Build history of the part. All positions in model axes, mm. Face numbers are marked on the shaded views. A direction names the side the tool comes from. Give positions to 0.01 mm unless a question says otherwise; leave off trailing zeros. Loops run counter-clockwise (first coordinate to the right, second up) from the corner with the lowest first, then second, coordinate; pieces in that order, holes last. Notation, with made-up numbers: (25.25, 39) - (29.25, 39) arc R20 cw to (29.25, 64) - close; hole circle Ø9 at (64.25, 30). An arc over 180 degrees is marked (long way). Return JSON: item names as keys, results as strings. Group by question number.
1) Slice it at A-A (z = 13.75). List the corners of the cut face in (x, y).
2) Slice it at D-D (y = 14). List the corners of the cut face in (x, z), and give its area (3 significant figures).
3) Slice it at C-C (y = -11). List the corners of the cut face in (x, z), and give its area (3 significant figures).
4) Drop flat-ended pins along their axis: pin 1 (6 mm diameter, centred on x = 0, z = 11, fed in from +Y); pin 2 (4 mm diameter, centred on x = 34.5, z = 5, fed in from -Y); pin 3 (7 mm diameter, centred on x = 28.5, z = 5.5, fed in from +Y). Give the stop position or say it passes through.
5) Drill centre lines: probe 1 along Y at (x, z) = (34.5, 2.5); probe 2 along X at (y, z) = (19, 1.25); probe 3 along Z at (x, y) = (-3, -24). Where is each one in solid material? Low to high. Write a range as from..to.
6) 3-axis set-ups, long thin cutter, end or side, ignore diameter. For the marked faces 1, 2, 3, 4 and 5: which of +Z, -Z, +X, -X, +Y, -Y reach the whole face in a straight line?
7) Slice it at B-B (x = -13). List the corners of the cut face in (y, z) (3 decimals), and give its area (4 significant figures).
8) Mould opens along X. For the marked faces 6, 7 and 8 say: released by +X, released by -X, zero draft, split by the parting line, or undercut.
```python
from build123d import *

# Parameters (mm, degrees)
F0_W      = 85
F0_H      = 56
F1_DEPTH  = 1.5
F2_R      = 2
F3_W      = 50
F3_H      = 5
F4_DEPTH  = 8.5
F5_W      = 17
F5_H      = 13.3
F5_W_2    = 20
F5_H_2    = 16
F6_DEPTH  = 14
F7_W      = 16
F7_H      = 14
F7_W_2    = 13.3
F8_DEPTH  = 2.38
F9_W      = 14
F9_H      = 14
F10_DEPTH = 1


with BuildPart() as f1:
    # F0 (on Top) → F1 (new body)
    with BuildSketch(Plane.XY):
        Rectangle(F0_W, F0_H)
    extrude(amount=F1_DEPTH)

    # F2
    f2_edges = [f1.edges().sort_by_distance(p)[0] for p in [
        (-42.5, -28, 0.75),
        (-42.5, 28, 0.75),
        (42.5, -28, 0.75),
        (42.5, 28, 0.75),
    ]]
    fillet(f2_edges, radius=F2_R)

    # F3 (on face) → F4 (join)
    with BuildSketch(Plane.XY.offset(1.5)):
        with Locations((-10.955842, 23.976474)):
            Rectangle(F3_W, F3_H)
    extrude(amount=F4_DEPTH)

    # F5 (on face) → F6 (join)
    with BuildSketch(Plane.XY.offset(1.5)):
        with Locations((34, 18.15)):
            Rectangle(F5_W, F5_H)
        with Locations((34, 0.85)):
            Rectangle(F5_W, F5_H)
        with Locations((32.5, -17.8)):
            Rectangle(F5_W_2, F5_H_2)
    extrude(amount=F6_DEPTH)

    # F7 (on face) → F8 (join)
    with BuildSketch(Plane.YZ.offset(42.5)):
        with Locations((-17.8, 8.5)):
            Rectangle(F7_W, F7_H)
        with Locations((0.85, 8.5)):
            Rectangle(F7_W_2, F7_H)
        with Locations((18.15, 8.5)):
            Rectangle(F7_W_2, F7_H)
    extrude(amount=F8_DEPTH)

    # F9 (on face) → F10 (join)
    with BuildSketch(Plane.XY.offset(1.5)):
        with Locations((-14.045779, 3.365002)):
            Rectangle(F9_W, F9_H)
    extrude(amount=F10_DEPTH)


solid = f1.part
```
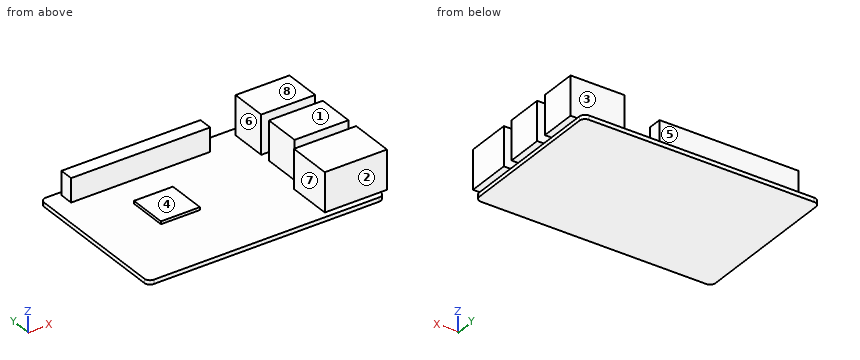
Results:
{
 "1": {"outline": "(22.5, -25.8) - (44.88, -25.8) - (44.88, -9.8) - (22.5, -9.8) - close; (25.5, -5.8) - (44.88, -5.8) - (44.88, 7.5) - (25.5, 7.5) - close; (25.5, 11.5) - (44.88, 11.5) - (44.88, 24.8) - (25.5, 24.8) - close"},
 "2": {"outline": "(-42.5, 0) - (42.5, 0) - (42.5, 1.5) - (44.88, 1.5) - (44.88, 15.5) - (25.5, 15.5) - (25.5, 1.5) - (-42.5, 1.5) - close", "area": "399 mm2"},
 "3": {"outline": "(-42.5, 0) - (42.5, 0) - (42.5, 1.5) - (44.88, 1.5) - (44.88, 15.5) - (22.5, 15.5) - (22.5, 1.5) - (-42.5, 1.5) - close", "area": "441 mm2"},
 "4": {"pin 1": "y = 26.48", "pin 2": "y = -25.8", "pin 3": "y = 24.8"},
 "5": {"probe 1": "-25.8..-9.8, -5.8..7.5, 11.5..24.8", "probe 2": "-42.5..42.5", "probe 3": "0..1.5"},
 "6": {"face 1": "+Z, +X, -X, +Y, -Y", "face 2": "+Z, +X, -X, -Y", "face 3": "+Z, +X, +Y", "face 4": "+Z, -X, -Y", "face 5": "+Z, +X, -X, +Y"},
 "7": {"outline": "(-28, 0) - (28, 0) - (28, 1.5) - (26.476, 1.5) - (26.476, 10) - (21.476, 10) - (21.476, 1.5) - (10.365, 1.5) - (10.365, 2.5) - (-3.635, 2.5) - (-3.635, 1.5) - (-28, 1.5) - close", "area": "140.5 mm2"},
 "8": {"face 6": "undercut", "face 7": "released by -X", "face 8": "zero draft"}
}
